from build123d import *

# Parameters (mm, degrees)
F0_R     = 0.8
F0_R_2   = 3.2
F0_R_3   = 1
F1_DEPTH = 6
F3_DEPTH = 6
F4_W     = 4.4655336533
F4_H     = 0.3993565915
F4_W_2   = 0.3993565915
F4_H_2   = 4.4655336533
F5_DEPTH = 4.5
F6_R     = 0.7
F7_DEPTH = 5
F8_DEPTH = 10


with BuildPart() as f1:
    # F0 (on Front) → F1 (new body)
    with BuildSketch(Plane.XZ):
        with BuildLine():
            Line((-7, -4.5), (7, -4.5))
            ThreePointArc((7, -4.5), (10.1819805153, -3.1819805153), (11.5, 0))
            ThreePointArc((11.5, 0), (10.1819805153, 3.1819805153), (7, 4.5))
            Line((7, 4.5), (-7, 4.5))
            ThreePointArc((-7, 4.5), (-10.1819805153, 3.1819805153), (-11.5, 0))
            ThreePointArc((-11.5, 0), (-10.1819805153, -3.1819805153), (-7, -4.5))
        make_face()
        with Locations((-9, 0)):
            Circle(F0_R, mode=Mode.SUBTRACT)
        Circle(F0_R_2, mode=Mode.SUBTRACT)
        with Locations((9, 0)):
            Circle(F0_R, mode=Mode.SUBTRACT)
        Circle(F0_R_2)
        Circle(F0_R_3, mode=Mode.SUBTRACT)
        Circle(F0_R_3)
        with Locations((9, 0)):
            Circle(F0_R)
        with Locations((-9, 0)):
            Circle(F0_R)
    extrude(amount=-F1_DEPTH)

    # F2 (on face) → F3 (join)
    with BuildSketch(Plane(origin=(0, 6, 0), x_dir=(-1, 0, 0), z_dir=(0, 1, 0))):
        with BuildLine():
            Line((7, 4.5), (-2.3691008836, 4.5))
            ThreePointArc((-2.3691008836, 4.5), (-5.1975280083, 3.3284271247), (-6.3691008836, 0.5))
            Line((-6.3691008836, 0.5), (-6.3691008836, -0.5))
            ThreePointArc((-6.3691008836, -0.5), (-5.1975280083, -3.3284271247), (-2.3691008836, -4.5))
            Line((-2.3691008836, -4.5), (7, -4.5))
            Line((7, -4.5), (7, 4.5))
        make_face()
    extrude(amount=F3_DEPTH)

    # F4 (on face) → F5 (join)
    with BuildSketch(Plane(origin=(0, 12, 0), x_dir=(-1, 0, 0), z_dir=(0, 1, 0))):
        with Locations((1.0412741685, 3.2637477852)):
            Rectangle(F4_W, F4_H)
        with Locations((1.0412741685, 0.8087011712)):
            Rectangle(F4_W, F4_H)
        with Locations((5.7582546142, -0.0916777644)):
            Rectangle(F4_W_2, F4_H_2)
    extrude(amount=F5_DEPTH)

    # F6 (on face) → F7 (cut)
    with BuildSketch(Plane.XY.offset(3.463426081)):
        with Locations((-1.0412741685, 14.6806975827)):
            Circle(F6_R)
    extrude(amount=-F7_DEPTH, mode=Mode.SUBTRACT)

    # F0 (on Front) → F8 (join)
    with BuildSketch(Plane.XZ):
        Circle(F0_R_2)
        Circle(F0_R_3, mode=Mode.SUBTRACT)
        Circle(F0_R_3)
    extrude(amount=F8_DEPTH)


solid = f1.part
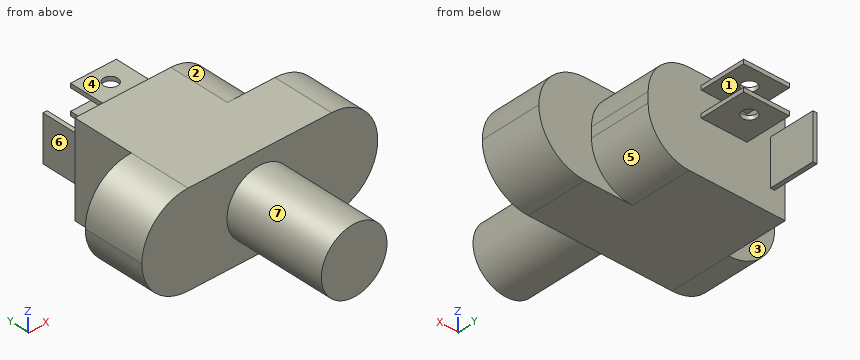
Could you check a few things on this model? Use its own coordinates, in mm. Face numbers are marked on the shaded views. A direction names the side the tool comes from. Round coordinates to 2 decimals unless told otherwise and drop trailing zeros. Write each loop counter-clockwise with the first axis right and the second up, starting at its lowest first coordinate (ties: lowest second). Pieces come first, ordered by that corner, then holes. Notation, with made-up numbers: (-26, 5.25) - (16, 5.25) arc R13 cw to (16, 12.25) - close; hole circle Ø4 at (63.5, -35.75). An arc over 180 degrees is marked (long way). Put each result on its own line as item: value. Start each with the question number.
(1) I want a section at D-D, the plane y = 4.5. Please give me the cut outline in (x, z), plus the area to 3 significant figures.
(2) Thinking about a two-plate mould opening in Z: for the marked faces 1, 2 and 3, which applies, released by +Z, released by -Z, zero draft, split by the parting line, or undercut?
(3) I want a section at C-C, the plane z = 2.75. Please give me the cut outline in (x, y), plus the area to 3 significant figures.
(4) For the marked faces 4, 5, 6 and 7, which set-ups out of +Z, -Z, +X, -X, +Y, -Y let a thin tool reach every point of the face, with its end or its side?
(5) I want a section at B-B, the plane y = 7.5. Please give me the cut outline in (x, z), plus the area to 3 significant figures.
(6) I want a section at A-A, the plane x = 0. Please give me the cut outline in (y, z).
(7) I need wall thicknesses on probe 1 along Y at (x, z) = (-9, 0.75); probe 2 along Y at (x, z) = (-4, -3); probe 3 along X at (y, z) = (3, 0.25). Which ranges of each line are inside material? Lowest first, please.
(8) Will these pins go through, and if not, where does the flat tip stop? pin 1 (3 mm diameter, centred on y = 9.5, z = 1, fed in from -X); pin 2 (5 mm diameter, centred on x = -1, y = 13.5, fed in from +Z); pin 3 (5 mm diameter, centred on x = 6.5, y = 13, fed in from -Z); pin 4 (3 mm diameter, centred on y = -0.5, z = 2, fed in from +X).
Here are the results:
1. outline: (-7, -4.5) - (7, -4.5) arc R4.5 ccw to (7, 4.5) - (-7, 4.5) arc R4.5 ccw to start
1. area: 190 mm^2
2. face 1: undercut
2. face 2: released by +Z
2. face 3: zero draft
3. outline: (-10.56, 0) - (-1.64, 0) - (-1.64, -10) - (1.64, -10) - (1.64, 0) - (10.56, 0) - (10.56, 6) - (5.68, 6) - (5.68, 12) - (-7, 12) - (-7, 6) - (-10.56, 6) - close
3. area: 236 mm^2
4. face 4: +Z, +X, -X, +Y
4. face 5: -Z, +X, +Y
4. face 6: +Z, -Z, -X, +Y
4. face 7: -Y
5. outline: (-7, -4.5) - (2.37, -4.5) arc R4 ccw to (6.37, -0.5) - (6.37, 0.5) arc R4 ccw to (2.37, 4.5) - (-7, 4.5) - close
5. area: 113 mm^2
6. outline: (-10, -3.2) - (0, -3.2) - (0, -4.5) - (12, -4.5) - (12, 0.61) - (16.5, 0.61) - (16.5, 1.01) - (12, 1.01) - (12, 3.06) - (16.5, 3.06) - (16.5, 3.46) - (12, 3.46) - (12, 4.5) - (0, 4.5) - (0, 3.2) - (-10, 3.2) - close
7. probe 1: y = 0 to 6
7. probe 2: y = 0 to 12
7. probe 3: x = -11.49 to 11.49
8. pin 1: stops at x = -7
8. pin 2: stops at z = 4.5
8. pin 3: stops at z = -4.05
8. pin 4: stops at x = 11.46
